```python
from build123d import *

# Parameters (mm, degrees)
F0_W     = 127
F0_H     = 76.2
F1_DEPTH = 3.175
F2_W     = 14.131395125
F2_H     = 3.175
F3_DEPTH = 25.4


# Not quite as in the source:
# - a length typed as a fraction of an inch, garbled in the dataset ("3 / 203.2 mm" for 3/8 in), is restored


with BuildPart() as f1:
    # F0 (on Top) → F1 (new body)
    with BuildSketch(Plane.XY):
        Polygon((84.1955885406, 47.9249996081), (65.1455885406, 47.9249996081), (65.1455885406, -28.2750003919), (84.1955885406, -28.2750003919), (103.2455885406, -15.5750003919), (103.2455885406, 35.2249996081), align=None)
        with Locations((1.6455885406, 9.8249996081)):
            Rectangle(F0_W, F0_H)
    extrude(amount=F1_DEPTH)

    # F2 (on face) → F3 (cut)
    with BuildSketch(Plane.XY.offset(3.175)):
        with Locations((89.8298909781, 33.6374996081)):
            Rectangle(F2_W, F2_H)
        with Locations((89.8298909781, -13.9875003919)):
            Rectangle(F2_W, F2_H)
    extrude(amount=-F3_DEPTH, mode=Mode.SUBTRACT)


solid = f1.part
```
Check sheet for the modelled part. Datum: model origin and axes. Units: mm. A direction names the side the tool comes from. Coordinates: 2 decimals unless noted, no trailing zeros. Write each loop counter-clockwise with the first axis right and the second up, starting at its lowest first coordinate (ties: lowest second). Pieces come first, ordered by that corner, then holes. Notation, with made-up numbers: M -15.5,43.25 L -11.5,43.25 A35 ccw -11.5,75.25 Z; hole C 80,49 d7. An arc over 180 degrees is marked long. Write item = value, one per line. Start each with the question number.
1. Go/stop test with flat-tipped pins: pin 1 (1.6 mm diameter, centred on x = 93, z = 1, fed in from +Y); pin 2 (1 mm diameter, centred on x = 90, z = 2, fed in from -Y); pin 3 (1 mm diameter, centred on x = 92.5, z = 2, fed in from -Y). Record where each tip stops, or that it passes through.
2. Sectioned sample at B-B (y = -18). Record the cut outline in (x, z) (3 decimals), then the cut area to 3 significant figures.
3. Sectioned sample at A-A (z = 1.8). Record the cut outline in (x, y) (3 decimals).
4. Tool access check on faces 4 (the flat face through (93.59, -22.01, 1.57)), 5 (the flat face through (96.896, 34, 2)). Record the directions out of +Z, -Z, +X, -X, +Y, -Y that give a thin tool (end or side, any length) a straight path to the whole face; none if there is none.
5. Mould release check, pull along X, two halves, no side actions. Record for faces 1 (the flat face through (10, -28.275, 2)), 2 (the flat face through (93.85, 41.49, 1.57)), 3 (the flat face through (96.896, -14, 2)): pulls with the +X half, pulls with the -X half, needs draft (parallel to the pull), parting line crosses it, or undercut.
6. Thickness scan on probe 1 along X at (y, z) = (-22, 0.75); probe 2 along X at (y, z) = (-24, 0.35). Record the ranges inside material, lowest first.
The answers:
q1.pin_1 = 42.59
q1.pin_2 = -24.74
q1.pin_3 = -23.07
q2.outline = M -61.854,0 L 99.608,0 L 99.608,3.175 L -61.854,3.175 Z
q2.area = 513 mm²
q3.outline = M -61.854,-28.275 L 84.196,-28.275 L 103.246,-15.575 L 103.246,35.225 L 84.196,47.925 L -61.854,47.925 Z; hole M 82.764,-15.575 L 96.896,-15.575 L 96.896,-12.4 L 82.764,-12.4 Z; hole M 82.764,32.05 L 96.896,32.05 L 96.896,35.225 L 82.764,35.225 Z
q4.face_4 = +Z, -Z, +X, -Y
q4.face_5 = +Z, -Z
q5.face_1 = needs draft
q5.face_2 = pulls with the +X half
q5.face_3 = undercut
q6.probe_1 = -61.85 to 93.61
q6.probe_2 = -61.85 to 90.61
